The listing builds one solid part. Answer for the finished solid, in the listing's coordinates (mm). Face numbers are marked on the shaded views. A direction names the side the tool comes from. Give positions to 0.01 mm unless a question says otherwise; leave off trailing zeros. Write each loop counter-clockwise with the first axis right and the second up, starting at its lowest first coordinate (ties: lowest second). Pieces come first, ordered by that corner, then holes. Notation, with made-up numbers: (48, 62.25) -> (77, 62.25) arc R13 cw to (77, 68.25) -> close; hole circle Ø10 at (29, -40). An arc over 180 degrees is marked (long way). One line per question, with ' | ' between items.
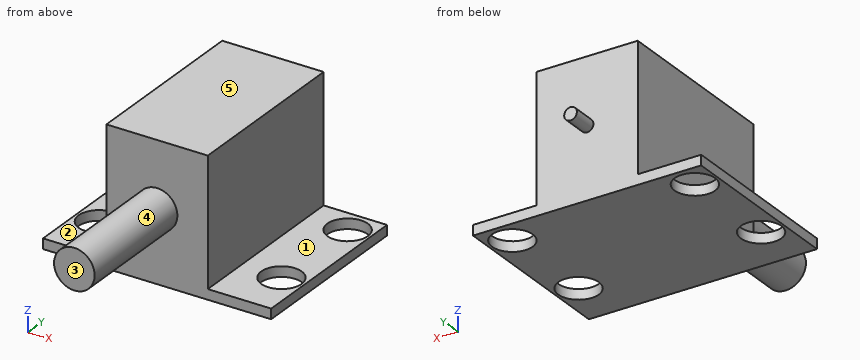
from build123d import *

# Parameters (mm, degrees)
SKETCH_1_W          = 45
SKETCH_1_H          = 35
EXTRUDE_1_DEPTH     = 2
SKETCH_2_W          = 20
SKETCH_2_H          = 35
EXTRUDE_2_DEPTH     = 25
SKETCH_3_R          = 4
EXTRUDE_3_DEPTH     = 25
SKETCH_4_R          = 1.25
EXTRUDE_4_DEPTH     = 5
SKETCH_5_R          = 4
CUT_EXTRUDE_1_DEPTH = 28


with BuildPart() as part:
    # ｽｹｯﾁ1 → ﾎﾞｽ - 押し出し1 (new body)
    with BuildSketch(Plane.XY):
        Rectangle(SKETCH_1_W, SKETCH_1_H)
    extrude(amount=EXTRUDE_1_DEPTH)

    # ｽｹｯﾁ2 → ﾎﾞｽ - 押し出し2 (add)
    with BuildSketch(Plane.XY.offset(2)):
        Rectangle(SKETCH_2_W, SKETCH_2_H)
    extrude(amount=EXTRUDE_2_DEPTH)

    # ｽｹｯﾁ3 → ﾎﾞｽ - 押し出し3 (add)
    with BuildSketch(Plane(origin=(0, -17.5, 0), x_dir=(-1, 0, 0), z_dir=(0, -1, 0))):
        with Locations((0, -14)):
            Circle(SKETCH_3_R)
    extrude(amount=EXTRUDE_3_DEPTH)

    # ｽｹｯﾁ4 → ﾎﾞｽ - 押し出し4 (add)
    with BuildSketch(Plane(origin=(0, 17.5, 0), x_dir=(1, 0, 0), z_dir=(0, 1, 0))):
        with Locations((0, -14)):
            Circle(SKETCH_4_R)
    extrude(amount=EXTRUDE_4_DEPTH)

    # ｽｹｯﾁ5 → ｶｯﾄ - 押し出し1 (cut, through all)
    with BuildSketch(Plane(origin=(0, 0, 0), x_dir=(-1, 0, 0), z_dir=(0, 0, -1))):
        with Locations((18, -7.5)):
            Circle(SKETCH_5_R)
        with Locations((18, 12.5)):
            Circle(SKETCH_5_R)
        with Locations((-18, 12.5)):
            Circle(SKETCH_5_R)
        with Locations((-18, -7.5)):
            Circle(SKETCH_5_R)
    extrude(amount=-CUT_EXTRUDE_1_DEPTH, mode=Mode.SUBTRACT)


solid = part.part
Item 1: Find section B-B (x = 18). Write down the section's boundary in (y, z), then the cut area to 3 significant figures.
Answers below:
outline: (-17.5, 0) -> (-11.5, 0) -> (-11.5, 2) -> (-17.5, 2) -> close; (-3.5, 0) -> (8.5, 0) -> (8.5, 2) -> (-3.5, 2) -> close; (16.5, 0) -> (17.5, 0) -> (17.5, 2) -> (16.5, 2) -> close | area: 38.0 mm²
Item 2: Flat-ended cylindrical pins translate along their axes: pin 1 (8 mm diameter, centred on y = -34, z = 17.5, fed in from +X); pin 2 (10 mm diameter, centred on x = 14, y = -5.5, fed in from +Z); pin 3 (12.5 mm diameter, centred on y = -1, z = 13, fed in from -X); pin 4 (3 mm diameter, centred on y = -20, z = 21.5, fed in from -X). Find the tip coordinate at first contact, or state that the pin passes through.
Answers below:
pin 1: x = 4 | pin 2: z = 27 | pin 3: x = -10 | pin 4: through
Item 3: Find section A-A (y = -7.5). Write down the section's boundary in (x, z), then the cut area to 3 significant figures.
Answers below:
outline: (-22.5, 0) -> (-22, 0) -> (-22, 2) -> (-22.5, 2) -> close; (-14, 0) -> (14, 0) -> (14, 2) -> (10, 2) -> (10, 27) -> (-10, 27) -> (-10, 2) -> (-14, 2) -> close; (22, 0) -> (22.5, 0) -> (22.5, 2) -> (22, 2) -> close | area: 558 mm²
Item 4: A tool of negligible diameter and unlimited length cuts with its end or side. For the marked faces 1, 2, 3, 4 and 5, from which of +Z, -Z, +X, -X, +Y, -Y can it reach the whole face along a straight path? Write none if from no direction.
Answers below:
face 1: +Z, +X, +Y, -Y | face 2: +Z, -X, +Y, -Y | face 3: +Z, -Z, +X, -X, -Y | face 4: -Y | face 5: +Z, +X, -X, +Y, -Y
Item 5: Consider line 1 (Y direction, x = 18, z = 0.7); line 2 (X direction, y = -2, z = 22.25); line 3 (Y direction, x = -3.5, z = 16.5). Determine where each line is inside the solid, lowest interval first. Write a range as [from, to].
Answers below:
line 1: [-17.5, -11.5], [-3.5, 8.5], [16.5, 17.5] | line 2: [-10, 10] | line 3: [-17.5, 17.5]
Item 6: Find section C-C (x = 0). Write down the section's boundary in (y, z).
Answers below:
outline: (-42.5, 10) -> (-17.5, 10) -> (-17.5, 0) -> (17.5, 0) -> (17.5, 12.75) -> (22.5, 12.75) -> (22.5, 15.25) -> (17.5, 15.25) -> (17.5, 27) -> (-17.5, 27) -> (-17.5, 18) -> (-42.5, 18) -> close
Item 7: Find section D-D (z = 14). Write down the section's boundary in (x, y).
Answers below:
outline: (-10, -17.5) -> (-4, -17.5) -> (-4, -42.5) -> (4, -42.5) -> (4, -17.5) -> (10, -17.5) -> (10, 17.5) -> (1.25, 17.5) -> (1.25, 22.5) -> (-1.25, 22.5) -> (-1.25, 17.5) -> (-10, 17.5) -> close
